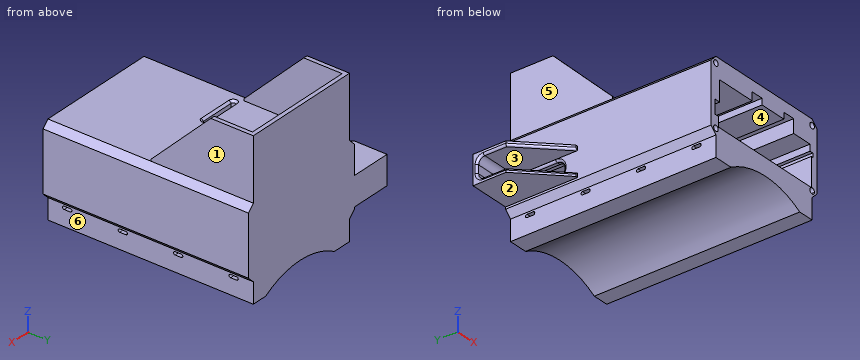
```python
from build123d import *

# Parameters (mm, degrees)
SKETCH043_W         = 65
SKETCH043_H         = 100
PAD_DEPTH           = 35
POCKET_DEPTH        = 96
CHAMFER_SIZE        = 3
SKETCH045_W         = 25
SKETCH045_H         = 25
POCKET001_DEPTH     = 10
CHAMFER001_SIZE     = 4
CHAMFER002_SIZE     = 3
CHAMFER003_SIZE     = 3
PAD001_DEPTH        = 30
CHAMFER004_SIZE     = 29
CHAMFER005_SIZE     = 3
SKETCH047_R         = 1.4
POCKET002_DEPTH     = 5
SKETCH048_W         = 59
SKETCH048_H         = 100
PAD002_DEPTH        = 10
SKETCH049_R         = 40
POCKET003_DEPTH     = 100
POCKET004_DEPTH     = 500
LINEARPATTERN_COUNT = 4
LINEARPATTERN_PITCH = 27
SKETCH051_R         = 1.4
POCKET005_DEPTH     = 10
POCKET006_DEPTH     = 11
CHAMFER006_SIZE     = 1
CHAMFER007_SIZE     = 1
CHAMFER008_SIZE     = 2
POCKET008_DEPTH     = 5
PAD005_DEPTH        = 20
CHAMFER010_SIZE     = 19
FILLET001_R         = 3
FILLET002_R         = 1
FILLET003_R         = 1


with BuildPart() as part:
    # Sketch043 → Pad (new body)
    with BuildSketch(Plane.XY):
        with Locations((-0.83, -1.54)):
            Rectangle(SKETCH043_W, SKETCH043_H)
    extrude(amount=PAD_DEPTH)

    # Sketch042 (on Face3 of Pad) → Pocket (cut)
    with BuildSketch(Plane.XZ.offset(51.54)):
        Polygon((0, 4.25), (-28.6, 4.25), (-28.6, 9.01), (-30.75, 9.01), (-30.75, 15.73), (-28.01, 15.73), (-28.01, 25.67), (-8.15, 25.67), (-8.15, 29.73), (-2.01, 29.73), (-2.01, 26.75), (11.35, 26.75), (11.35, 29.82), (17.4, 29.82), (17.4, 23.21), (27.42, 23.21), (27.42, 20.07), (29.09, 20.07), (29.09, 18.12), (28.23, 18.12), (28.23, 4.25), align=None)
    extrude(amount=-POCKET_DEPTH, mode=Mode.SUBTRACT)

    # Chamfer
    chamfer_edges = [part.edges().sort_by_distance(p)[0] for p in [
        (-33.33, -1.54, 35),
        (-33.33, -1.54, 0),
        (31.67, -1.54, 35),
        (31.67, -1.54, 0),
    ]]
    chamfer(chamfer_edges, length=CHAMFER_SIZE)

    # Sketch045 (on Face6 of Chamfer) → Pocket001 (cut)
    with BuildSketch(Plane.XY.offset(35)):
        with Locations((4.82, 15.27)):
            Rectangle(SKETCH045_W, SKETCH045_H)
    extrude(amount=-POCKET001_DEPTH, mode=Mode.SUBTRACT)

    # Chamfer001
    chamfer001_edges = [part.edges().sort_by_distance(p)[0] for p in [
        (4.82, 2.77, 35),
    ]]
    chamfer(chamfer001_edges, length=CHAMFER001_SIZE)

    # Chamfer002
    chamfer002_edges = [part.edges().sort_by_distance(p)[0] for p in [
        (-7.68, 15.27, 35),
    ]]
    chamfer(chamfer002_edges, length=CHAMFER002_SIZE)

    # Chamfer003
    chamfer003_edges = [part.edges().sort_by_distance(p)[0] for p in [
        (17.32, 15.27, 35),
    ]]
    chamfer(chamfer003_edges, length=CHAMFER003_SIZE)

    # Sketch046 (on Face1 of Chamfer003) → Pad001 (join)
    with BuildSketch(Plane.XY.offset(35)):
        Polygon((-30.33, 48.46), (28.67, 48.46), (28.67, -1.23), (26.67, -1.23), (26.67, 46.46), (-28.33, 46.46), (-28.33, -1.23), (-30.33, -1.23), align=None)
    extrude(amount=PAD001_DEPTH)

    # Chamfer004
    chamfer004_edges = [part.edges().sort_by_distance(p)[0] for p in [
        (-29.33, -1.23, 65),
        (27.67, -1.23, 65),
    ]]
    chamfer(chamfer004_edges, length=CHAMFER004_SIZE)

    # Chamfer005
    chamfer005_edges = [part.edges().sort_by_distance(p)[0] for p in [
        (4.67, 2.77, 26.75),
    ]]
    chamfer(chamfer005_edges, length=CHAMFER005_SIZE)

    # Sketch047 (on Face6 of Chamfer005) → Pocket002 (cut)
    with BuildSketch(Plane.XZ.offset(51.54)):
        with Locations((-30.33, 32)):
            Circle(SKETCH047_R)
        with Locations((-30.33, 3)):
            Circle(SKETCH047_R)
        with Locations((28.67, 32)):
            Circle(SKETCH047_R)
        with Locations((28.67, 3)):
            Circle(SKETCH047_R)
    extrude(amount=-POCKET002_DEPTH, mode=Mode.SUBTRACT)

    # Sketch048 (on Face19 of Pocket002) → Pad002 (join)
    with BuildSketch(Plane(origin=(0, 0, 0), x_dir=(1, 0, 0), z_dir=(0, 0, -1))):
        with Locations((-0.83, 1.54)):
            Rectangle(SKETCH048_W, SKETCH048_H)
    extrude(amount=PAD002_DEPTH)

    # Sketch049 (on Face19 of Pad002) → Pocket003 (cut)
    with BuildSketch(Plane.XZ.offset(51.54)):
        with Locations((0, -44)):
            Circle(SKETCH049_R)
    extrude(amount=-POCKET003_DEPTH, mode=Mode.SUBTRACT)

    # Sketch050 (on Face53 of Pocket003) → Pocket004 (cut)
    with BuildSketch(Plane(origin=(-30.33, 0, 0), x_dir=(0, -1, 0), z_dir=(-1, 0, 0))):
        with BuildLine():
            ThreePointArc((-40.389904, -0.843272), (-41.139904, -1.593272), (-40.389904, -2.343272))
            Line((-40.389904, -2.343272), (-37.389904, -2.343272))
            ThreePointArc((-37.389904, -2.343272), (-36.639904, -1.593272), (-37.389904, -0.843272))
            Line((-40.389904, -0.843272), (-37.389904, -0.843272))
        make_face()
    pocket004 = extrude(amount=-POCKET004_DEPTH, mode=Mode.SUBTRACT)

    # LinearPattern: Pocket004 ×4
    with Locations(*[(0, -i * LINEARPATTERN_PITCH, 0) for i in range(1, LINEARPATTERN_COUNT)]):
        add(pocket004, mode=Mode.SUBTRACT)

    # Sketch051 (on Face20 of LinearPattern) → Pocket005 (cut)
    with BuildSketch(Plane.XY.offset(35)):
        with Locations((-10.33, 32.46)):
            Circle(SKETCH051_R)
    extrude(amount=-POCKET005_DEPTH, mode=Mode.SUBTRACT)

    # Sketch052 (on Face20 of Pocket005) → Pocket006 (cut)
    with BuildSketch(Plane.XY.offset(35)):
        with BuildLine():
            ThreePointArc((-25.13, -3.04), (-26.13, -4.04), (-25.13, -5.04))
            Line((-25.13, -5.04), (-8.13, -5.04))
            ThreePointArc((-8.13, -5.04), (-7.13, -4.04), (-8.13, -3.04))
            Line((-25.13, -3.04), (-8.13, -3.04))
        make_face()
    extrude(amount=-POCKET006_DEPTH, mode=Mode.SUBTRACT)

    # Chamfer006
    chamfer006_edges = [part.edges().sort_by_distance(p)[0] for p in [
        (-16.63, -3.04, 35),
    ]]
    chamfer(chamfer006_edges, length=CHAMFER006_SIZE)

    # Chamfer007
    chamfer007_edges = [part.edges().sort_by_distance(p)[0] for p in [
        (-16.64, -5.04, 25.67),
    ]]
    chamfer(chamfer007_edges, length=CHAMFER007_SIZE)

    # Chamfer008
    chamfer008_edges = [part.edges().sort_by_distance(p)[0] for p in [
        (-8.15, -5.04, 28.2),
    ]]
    chamfer(chamfer008_edges, length=CHAMFER008_SIZE)

    # Sketch056 (on Face24 of Chamfer008) → Pocket008 (cut)
    with BuildSketch(Plane(origin=(-33.33, 0, 0), x_dir=(0, -1, 0), z_dir=(-1, 0, 0))):
        with BuildLine():
            ThreePointArc((-38, 14.96), (-42, 10.96), (-38, 6.96))
            Line((-38, 6.96), (-24, 6.96))
            ThreePointArc((-24, 6.96), (-20, 10.96), (-24, 14.96))
            Line((-38, 14.96), (-24, 14.96))
        make_face()
    extrude(amount=-POCKET008_DEPTH, mode=Mode.SUBTRACT)

    # Sketch057 (on Face24 of Pocket008) → Pad005 (join)
    with BuildSketch(Plane(origin=(-33.33, 0, 0), x_dir=(0, -1, 0), z_dir=(-1, 0, 0))):
        Polygon((-48.46, 18), (-13.46, 18), (-13.46, 16), (-46.46, 16), (-46.46, 6), (-13.46, 6), (-13.46, 4), (-48.46, 4), align=None)
    extrude(amount=PAD005_DEPTH)

    # Chamfer010
    chamfer010_edges = [part.edges().sort_by_distance(p)[0] for p in [
        (-53.33, 13.46, 5),
        (-53.33, 13.46, 17),
    ]]
    chamfer(chamfer010_edges, length=CHAMFER010_SIZE)

    # Fillet001
    fillet001_edges = [part.edges().sort_by_distance(p)[0] for p in [
        (-43.33, 46.46, 6),
        (-43.33, 46.46, 16),
    ]]
    fillet(fillet001_edges, radius=FILLET001_R)

    # Fillet002
    fillet002_edges = [part.edges().sort_by_distance(p)[0] for p in [
        (-53.33, 37.96, 16),
        (-43.83, 22.96, 16),
        (-43.83, 22.96, 6),
    ]]
    fillet(fillet002_edges, radius=FILLET002_R)

    # Fillet003
    fillet003_edges = [part.edges().sort_by_distance(p)[0] for p in [
        (-33.33, 20, 10.96),
    ]]
    fillet(fillet003_edges, radius=FILLET003_R)


with BuildPart() as part_1:
    # Body012 placement: moved
    add(part.part.moved(Location((0, 0, -8.6))))


solid = part_1.part
```
Can you work these out from the model? Positions are in its coordinate system, mm. Face numbers are marked on the shaded views. A direction names the side the tool comes from. Round coordinates to 2 decimals unless told otherwise and drop trailing zeros. Loops run counter-clockwise (first coordinate to the right, second up) from the corner with the lowest first, then second, coordinate; pieces in that order, holes last.
Item 1: If we mould it in two halves opening along Z, with no side actions, what happens to the marked faces 1, 2 and 3? For each: +Z half, -Z half, draft (parallel to the pull), parting line (faces both ways), or undercut.
Item 2: Suppose I cut it at C-C, the plane z = 42. Write out the boundary of the cut face in (x, y).
Item 3: Please list where these lines run through material, in increasing order: L1, parallel to X at y = -49.5, z = 23.4; L2, parallel to Y at x = -10, z = 24; L3, parallel to X at y = -39.5, z = 2.
Item 4: Will these pins go through, and if not, where does the flat tip stop? pin 1 Ø2.5 at (x, y) = (11.5, -14.5) entering from -Z; pin 2 Ø0.8 at (x, z) = (-34, -3.5) entering from -Y; pin 3 Ø0.5 at (x, z) = (-29, 27) entering from -Y.
Item 5: Suppose I cut it at A-A, the plane x = 4. State how many separate pieces and enclosed holes the cut face has, then the cut area to 3 significant figures.
Item 6: Which directions (+Z, -Z, +X, -X, +Y, -Y) give clear straight access to the entire face, cutting with the end or side of a thin tool? Please do the marked faces 4, 5 and 6.
Reported:
1. face 1: draft
1. face 2: -Z half
1. face 3: undercut
2. outline: (-30.33, 13.37) - (-28.33, 13.37) - (-28.33, 46.46) - (26.67, 46.46) - (26.67, 13.37) - (28.67, 13.37) - (28.67, 48.46) - (-30.33, 48.46) - close
3. L1: x = -33.33 to -31.73, -28.93 to 27.27, 30.07 to 31.67
3. L2: y = -51.54 to -5.04, -3.04 to 31.1, 33.82 to 48.46
3. L3: x = -33.33 to -30.75, 28.23 to 31.67
4. pin 1: stops at z = -14.69
4. pin 2: stops at y = 13.46
4. pin 3: stops at y = -1.23
5. separate pieces: 2
5. enclosed holes: 4
5. area: 1,580 mm2
6. face 4: -Y
6. face 5: +Z, -X, +Y, -Y
6. face 6: -Z, +X, +Y, -Y
